Autodesk Fusion 360 part; units mm, degrees
sketch "Sketch1" plane through (0, 0, 0) normal (0, 0, 1) x (1, 0, 0)
  line L0 (0, 0) -> (18, 0)
  line L1 (18, 0) -> (18, 18)
  line L2 (18, 18) -> (0, 18)
  line L3 (0, 18) -> (0, 0)
  line L4 (0, 18) -> (-10, 18)
  line L5 (-10, 18) -> (-10, 28)
  line L6 (-10, 28) -> (28, 28)
  line L7 (28, 28) -> (28, -10)
  line L8 (28, -10) -> (-10, -10)
  line L9 (-10, -10) -> (-10, 28)
  dimension "d1" = 18
  dimension "d2" = 18
  dimension "d3" = 10
  dimension "d4" = 10
  dimension "d5" = 10
  dimension "d6" = 10
extrude "Extrude1" add sketch "Sketch1" along normal blind 2
extrude "Extrude2" add sketch "Sketch1" along normal blind 1.8 contours L0 L1 L2 L3
sketch "Sketch2" plane through (0, -10, 0) normal (0, -1, 0) x (1, 0, 0)
  line L0 (-10, 0) -> (28, 0)
  line L1 (28, 0) -> (28, 2)
  line L2 (28, 2) -> (-10, 2)
  line L3 (-10, 2) -> (-10, 0)
  line L4 (9, 2) -> (-2.75, 2)
  line L5 (9, 2) -> (20.75, 2)
  line L6 (-2.75, 2) -> (-2.75, 0)
  line L7 (20.75, 2) -> (20.75, 0)
  dimension "d11" = 11.75
  dimension "d12" = 11.75
extrude "Extrude3" add sketch "Sketch2" along normal blind 30 contours L0 L2 L4 L5 L6 L7
sketch "Sketch3" plane through (0, 0, 2) normal (0, 0, 1) x (-1, 0, 0)
  line L0 (0, 0) -> (0, -18)
  line L1 (0, -18) -> (-18, -18)
  line L2 (-18, -18) -> (-18, 0)
  line L3 (-18, 0) -> (0, 0)
  line L4 (10, 10) -> (2.75, 10)
  line L5 (2.75, 10) -> (2.75, 40)
  line L6 (2.75, 40) -> (-20.75, 40)
  line L7 (-20.75, 40) -> (-20.75, 10)
  line L8 (-20.75, 10) -> (-28, 10)
  line L9 (-28, 10) -> (-28, -28)
  line L10 (-28, -28) -> (10, -28)
  line L11 (10, -28) -> (10, 10)
  line L12 (-9, 40) -> (-9, 0)
  line L13 (-31.221, 25) -> (-24.871, 25)
  line L14 (-9, 40) -> (-20.75, 40)
  line L15 (-9, 40) -> (2.75, 40)
  line L16 (0, 0) -> (0, 40)
  line L17 (0, 40) -> (-6.7, 40)
  line L18 (-6.7, 40) -> (-6.7, 0)
  line L19 (-18, 0) -> (-18, 40)
  line L20 (-11.3, 40) -> (-11.3, 0)
  line L21 (-18, 40) -> (-11.3, 40)
  dimension "d15" = 6.35
  dimension "d18" = 6.7
extrude "Extrude4" cut sketch "Sketch3" against normal blind 0.2 contours L3 L6 L15 L16 L17 L18 | L3 L6 L14 L19 L20 L21
chamfer "Chamfer1" distance 0.8 distance2 7 2 edges at (14.65, -40, 1.8) (3.35, -40, 1.8) measured on face at (8.2333, -40, 0.6) measured on face at (8.2333, -40, 0.6)
fillet "Fillet1" radius 7.5 2 edges at (-10, 28, 1) (28, 28, 1)
sketch "Sketch4" plane through (0, 0, 2) normal (0, 0, 1) x (-1, 0, 0)
  arc A0 (-28, -20.5) -> (-20.5, -28) centre (-20.5, -20.5) ccw
  line L0 (-20.5, -28) -> (2.5, -28)
  arc A1 (2.5, -28) -> (10, -20.5) centre (2.5, -20.5) ccw
  line L1 (10, -20.5) -> (10, 10)
  line L2 (10, 10) -> (2.75, 10)
  line L3 (2.75, 10) -> (2.75, 40)
  line L4 (2.75, 40) -> (0, 40)
  line L5 (0, 40) -> (0, -18)
  line L6 (0, -18) -> (-18, -18)
  line L7 (-18, -18) -> (-18, 40)
  line L8 (-18, 40) -> (-20.75, 40)
  line L9 (-20.75, 40) -> (-20.75, 10)
  line L10 (-20.75, 10) -> (-28, 10)
  line L11 (-28, 10) -> (-28, -20.5)
  line L12 (0, -18) -> (10, -18)
  line L13 (5, -18) -> (5, 0)
  line L14 (5, 0) -> (3, 0)
  line L15 (3, 0) -> (3, -18)
  line L16 (5, 0) -> (7, 0)
  line L17 (7, 0) -> (7, -18)
  line L18 (-9, -18) -> (-9, -9)
  line L19 (-25, 0) -> (-25, -18)
  line L20 (-23, -18) -> (-23, 0)
  line L21 (-21, 0) -> (-21, -18)
  line L22 (-18, -18) -> (-28, -18)
  line L23 (-23, 0) -> (-21, 0)
  line L24 (-23, 0) -> (-25, 0)
  line L25 (-18, -18) -> (0, 0)
  line L26 (0, -21) -> (-18, -21)
  line L27 (-18, -23) -> (0, -23)
  line L28 (0, -25) -> (-18, -25)
  line L29 (-18, -18) -> (-18, -28)
  line L30 (0, -23) -> (0, -21)
  line L31 (0, -23) -> (0, -25)
  dimension "d25" = 2
  dimension "d26" = 2
extrude "Extrude5" cut sketch "Sketch4" against normal blind 0.6 contours L19 L20 L22 L24 | L27 L28 L29 L31 | L20 L21 L22 L23 | L26 L27 L29 L30 | L12 L13 L16 L17 | L12 L13 L14 L15
Design review of the part built by this model. Coordinates are the model's own, in mm. A direction names the side the tool comes from. Coordinates: 2 decimals unless noted, no trailing zeros. Order: outer loops, then holes, each group sorted by start corner. A loop starts at its lowest first (then second) coordinate and runs counter-clockwise, first axis right, second up. Notation, with made-up numbers: (-32.75, -2) - (-14.75, -2) arc R18 ccw to (-14.75, 7) - close; hole circle Ø7 at (73, 2). An arc over 180 degrees is marked (long way). Answer in a Markdown table with one row per item.
(1) The part is to be moulded in two halves that separate along Y. For faces 6 (the flat face through (9, 28, 1)), 7 (the flat face through (28, 5, 1)), 8 (the flat face through (14.6, -36.5, 1.4)), 9 (the flat face through (-5, 9, 1.4)), say which applies: released by +Y, released by -Y, zero draft, split by the parting line, or undercut.
Checked values:
| item | result |
|---|---|
| face 6 | released by +Y |
| face 7 | zero draft |
| face 8 | released by -Y |
| face 9 | undercut |
(2) Clearance check with flat-ended pins moving along their axes: pin 1 (0.7 mm diameter, centred on x = 23.5, z = 1.5, fed in from -Y); pin 2 (0.7 mm diameter, centred on y = 22.5, z = 1.5, fed in from +X); pin 3 (0.8 mm diameter, centred on y = -21, z = 1.5, fed in from -X). State where each tip first meets the part, or that it passes through.
Checked values:
| item | result |
|---|---|
| pin 1 | y = -10 |
| pin 2 | x = 27.82 |
| pin 3 | x = -2.75 |
(3) Consider section C-C on y = 5. State the section outline as (x, z) points, plus the area to 3 significant figures.
Checked values:
| item | result |
|---|---|
| outline | (-10, 0) - (28, 0) - (28, 2) - (25, 2) - (25, 1.4) - (21, 1.4) - (21, 2) - (18, 2) - (18, 1.8) - (0, 1.8) - (0, 2) - (-3, 2) - (-3, 1.4) - (-7, 1.4) - (-7, 2) - (-10, 2) - close |
| area | 67.6 mm^2 |
(4) For faces 1 (the flat face through (-10, 5, 1)), 2 (the flat face through (3.3, -36.5, 1.4)), 3 (the flat face through (-6, -10, 1)), 4 (the flat face through (23, 9, 1.4)), 5 (the flat face through (24, -10, 1)), list the 3-axis set-ups (+Z, -Z, +X, -X, +Y, -Y) from which the entire face can be reached by the end or side of a thin tool; tool diameter is ignored.
Checked values:
| item | result |
|---|---|
| face 1 | +Z, -Z, -X, +Y, -Y |
| face 2 | +Z, -Y |
| face 3 | +Z, -Z, -X, -Y |
| face 4 | +Z |
| face 5 | +Z, -Z, +X, -Y |
(5) Consider section B-B on x = 12.5. State the section outline as (y, z) points, plus the area to 3 significant figures.
Checked values:
| item | result |
|---|---|
| outline | (-40, 0) - (28, 0) - (28, 2) - (25, 2) - (25, 1.4) - (21, 1.4) - (21, 2) - (18, 2) - (18, 1.8) - (-33, 1.8) - (-40, 1) - close |
| area | 119 mm^2 |
(6) Consider section A-A on y = -20.5. State the section outline as (x, z) points.
Checked values:
| item | result |
|---|---|
| outline | (-2.75, 0) - (20.75, 0) - (20.75, 2) - (18, 2) - (18, 1.8) - (11.3, 1.8) - (11.3, 2) - (6.7, 2) - (6.7, 1.8) - (0, 1.8) - (0, 2) - (-2.75, 2) - close |
(7) Wall thickness on line 1 along X through (y, z) = (5.5, 1.6); line 2 along Z through (x, y) = (15, 9); line 3 along X through (y, z) = (-30.5, 0.2): over which ranges is each line inside the solid? List them lowest first. Write a range as from..to.
Checked values:
| item | result |
|---|---|
| line 1 | -10..-7, -3..21, 25..28 |
| line 2 | 0..1.8 |
| line 3 | -2.75..20.75 |
(8) Consider section D-D on x = 22. State the section outline as (y, z) points.
Checked values:
| item | result |
|---|---|
| outline | (-10, 0) - (27.85, 0) - (27.85, 2) - (18, 2) - (18, 1.4) - (0, 1.4) - (0, 2) - (-10, 2) - close |
